CAD build for the part. Positions are in the model's coordinates, mm. Face numbers are marked on the shaded views. A direction names the side the tool comes from. Round coordinates to 2 decimals unless told otherwise and drop trailing zeros. Loops run counter-clockwise (first coordinate to the right, second up) from the corner with the lowest first, then second, coordinate; pieces in that order, holes last.
Autodesk Inventor part; units mm, degrees
ref_plane "РабПлоскость1" through (35, -50, -45) normal (0, 0, 1) x (1, 0, 0)
ref_plane "РабПлоскость2" through (-5, 20, -30) normal (0, 0, 1) x (1, 0, 0)
sketch "Эскиз1" plane through (0, 0, 0) normal (1, 0, 0) x (0, 1, 0)
  line L0 (-50, 80) -> (-50, 0)
  line L1 (-50, 0) -> (0, 0)
  line L2 (0, 0) -> (0, -30)
  line L3 (0, -30) -> (20, -30)
  line L4 (20, -30) -> (20, -45)
  line L5 (20, -45) -> (60, -45)
  line L6 (60, -45) -> (60, -30)
  arc A0 (60, -30) -> (-50, 80) centre (-50, -30) ccw
  line L7 (20, -30) -> (60, -30)
  dimension "d1" = 50
  dimension "d2" = 80
  dimension "d5" = 30
  dimension "d6" = 20
  dimension "d7" = 15
  dimension "d8" = 40
extrude "Выдавливание1" add sketch "Эскиз1" along normal mid plane 10 contours A0 L7 L3 L2 L1 L0
fillet "Сопряжение1" radius 5 2 edges at (0, 0, 0) (0, 0, -30)
sketch "Эскиз4" plane through (5, 0, 0) normal (1, 0, 0) x (0, 0, -1)
  arc A0 (30, 60) -> (-80, -50) centre (30, -50) ccw
  line L0 (-80, -50) -> (-50, -50)
  line L1 (-80, -50) -> (0, -50)
  arc A1 (-20, 12.44998) -> (-50, -50) centre (30, -50) ccw
  line L2 (-20, 12.44998) -> (-60.553851, 12.44998)
  line L3 (-20, -37.5) -> (-20, -62.5)
  line L4 (-20, 12.44998) -> (-20, 47.97959)
  point P0 (0, 0)
  point P1 (-20, -50)
  dimension "d16" = 30
  dimension "d19" = 25
  dimension "d20" = 30
sketch "Эскиз4 outline for Вращение2" plane through (5, 0, 0) normal (1, 0, 0) x (0, 0, -1)
  arc A0 (-50, -50) -> (-20, 12.44998) centre (30, -50) cw
  line L0 (-20, 12.44998) -> (-20, 47.97959)
  arc A1 (-20, 47.97959) -> (-80, -50) centre (30, -50) ccw
  line L1 (-80, -50) -> (-50, -50)
revolve "Вращение2" add sketch "Эскиз4 outline for Вращение2" angle 90 about axis through (5, -37.5, 20) along (0, 1, 0)
ref_plane "РабПлоскость1" through (35, -50, -45) normal (0, 0, 1) x (1, 0, 0)
ref_plane "РабПлоскость2" through (-5, 20, -30) normal (0, 0, 1) x (1, 0, 0)
sketch "Эскиз24" plane through (5, 60, -30) normal (0, 0, -1) x (-1, 0, 0)
  arc A0 (-20, 0) -> (-60, -40) centre (-20, -40) ccw
  line L0 (10, 0) -> (0, 0)
  line L1 (0, 0) -> (-20, 0)
  line L2 (-60, -40) -> (-60, -110)
  line L3 (-60, -110) -> (0, -110)
  line L4 (0, -55) -> (0, 0)
  line L5 (0, -110) -> (0, 0)
sketch "Эскиз18" plane through (5, 12.44998, 20) normal (0, 0, -1) x (-1, 0, 0)
  arc A0 (0, 35.52961) -> (-60, -62.44998) centre (50, -62.44998) ccw
  line L0 (-60, -62.44998) -> (-30, -62.44998)
  arc A1 (0, 0) -> (-30, -62.44998) centre (50, -62.44998) ccw
  line L1 (0, 35.52961) -> (0, 0)
  point P0 (5, -12.44998)
sketch "Эскиз19" plane through (5, 0, 0) normal (1, 0, 0) x (0, 0, -1)
  arc A0 (30, 60) -> (-20, 47.97959) centre (30, -50) ccw
  point P0 (0, 0)
ref_plane "РабПлоскость3" through (75, 0, 0) normal (1, 0, 0) x (0, 0, -1)
sketch "Эскиз23" plane through (75, 0, 0) normal (1, 0, 0) x (0, 0, -1)
  line L0 (40, -50) -> (-60, -50)
  point P0 (0, 0)
  point P1 (-20, -50)
  dimension "d111" = 100
  dimension "d112" = 40
sketch "Эскиз16" plane through (-5, 5, -30) normal (0, 0, -1) x (-1, 0, 0)
  line L0 (0, 0) -> (-10, 0)
  line L1 (0, 55) -> (0, 0)
  line L2 (0, 55) -> (-10, 55)
  line L3 (-10, 0) -> (-10, 18.536525)
  line L4 (-10, 55) -> (-30, 55)
  arc A0 (-30, 55) -> (-70, 15) centre (-30, 15) ccw
  line L5 (-70, 15) -> (-70, -55)
  line L6 (-70, -55) -> (-10, -55)
  line L7 (-10, -55) -> (-10, 0)
  point P0 (-5, -5)
sketch "Эскиз25" plane through (-5, -50, 0) normal (0, -1, 0) x (1, 0, 0)
  line L0 (0, -30) -> (0, -45)
  line L1 (0, -45) -> (42, -45)
  line L2 (42, -45) -> (42, 51)
  line L3 (42, 51) -> (0, 51)
  line L4 (0, 51) -> (0, -45)
  point P0 (5, 0)
  dimension "d124" = 42
  dimension "d125" = 96
sketch "Эскиз26" plane through (-5, 0, 0) normal (-1, 0, 0) x (0, 0, 1)
  line L0 (-36.339746, 50) -> (-36.339746, 30)
  line L1 (-45, 45) -> (-36.339746, 50)
  line L2 (-36.339746, 30) -> (-45, 35)
  line L3 (-45, 20) -> (-45, 60)
  circle A0 centre (15, -35) radius 5
  point P0 (0, 0)
sketch "Эскиз27" plane through (-5, 5, -45) normal (0, 0, -1) x (-1, 0, 0)
  line L0 (-62.5, -48) -> (-60, -55)
  line L1 (-47.5, -48) -> (-62.5, -48)
  line L2 (-50, -55) -> (-47.5, -48)
  line L3 (-70, -55) -> (0, -55)
  point P0 (-5, -5)
properties part number "Уголок_передней_крышки_2.0"
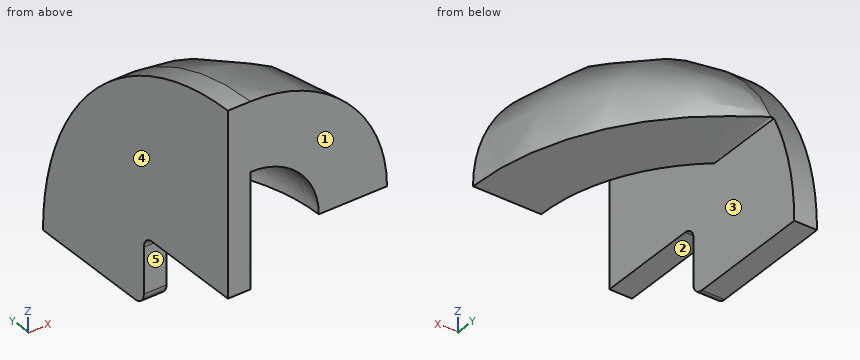
Item 1: Mould opens along X. For the marked faces 3, 4 and 5 say: released by +X, released by -X, zero draft, split by the parting line, or undercut.
Verdict:
face 3: undercut
face 4: released by -X
face 5: zero draft
Item 2: 3-axis set-ups, long thin cutter, end or side, ignore diameter. For the marked faces 1 and 2: which of +Z, -Z, +X, -X, +Y, -Y reach the whole face in a straight line?
Verdict:
face 1: +Z, -Z, +X, -X, -Y
face 2: -Z, +X, -X, -Y
Item 3: Cut at A-A (z = 1.5). List the corners of the cut face in (x, y).
Verdict:
outline: (-5, -50) - (5, -50) - (5, 55.39) - (-5, 55.39) - close
Item 4: Flat gauge pins, fed straight in: P1, Ø12, axis at x = 42.5, y = -1.5, coming from the -Z side; P2, Ø3, axis at x = -2.5, z = -10.5, coming from the -Y side; P3, Ø2, axis at x = 48.5, z = 64, coming from the -Y side; P4, Ø8, axis at x = 2.5, y = -26.5, coming from the -Z side. Where does each tip first touch, or does it go through?
Verdict:
P1: stops at z = 20
P2: stops at y = 0
P3: passes through
P4: stops at z = 0
